CAD build for the part. Positions are in the model's coordinates, mm. A direction names the side the tool comes from. Coordinates: 2 decimals unless noted, no trailing zeros. Loops run counter-clockwise (first coordinate to the right, second up) from the corner with the lowest first, then second, coordinate; pieces in that order, holes last. Notation, with made-up numbers: M -21,0 L -4,0 A21 cw -4,4 Z; hole C 57,6.25 d5. An arc over 180 degrees is marked long. Answer as a JSON object with one key per item and string values. Group by question number.
```python
from build123d import *

# Parameters (mm, degrees)
SKETCH_1_R          = 12.2
EXTRUDE_1_DEPTH     = 18.1
FILLET_1_R          = 2
SKETCH_2_R          = 12.5
EXTRUDE_2_DEPTH     = 19
SKETCH_3_R          = 3.5
EXTRUDE_3_DEPTH     = 2.5
SKETCH_4_R          = 1.5
EXTRUDE_4_DEPTH     = 9
CUT_EXTRUDE_1_DEPTH = 8
SKETCH_6_R          = 2.25
CUT_EXTRUDE_2_DEPTH = 1.5
SKETCH_8_R          = 1.5
CUT_EXTRUDE_3_DEPTH = 6
SKETCH_9_R          = 3.25
EXTRUDE_5_DEPTH     = 2
SKETCH_10_W         = 3
SKETCH_10_H         = 0.5
EXTRUDE_6_DEPTH     = 4


with BuildPart() as part:
    # 草图1 → 凸台-拉伸1 (new body)
    with BuildSketch(Plane.XY):
        with Locations(Location((0, 0, 0), (0, 0, 180))):
            Circle(SKETCH_1_R)
    extrude(amount=EXTRUDE_1_DEPTH)

    # 圆角1
    fillet_1_edges = [part.edges().sort_by_distance(p)[0] for p in [
        (12.2, 0, 18.1),
    ]]
    fillet(fillet_1_edges, radius=FILLET_1_R)

    # 草图2 → 凸台-拉伸2 (add)
    with BuildSketch(Plane.XY.offset(18.1)):
        Circle(SKETCH_2_R)
    extrude(amount=EXTRUDE_2_DEPTH)

    # 草图3 → 凸台-拉伸3 (add)
    with BuildSketch(Plane.XY.offset(37.1)):
        Circle(SKETCH_3_R)
    extrude(amount=EXTRUDE_3_DEPTH)

    # 草图4 → 凸台-拉伸4 (add)
    with BuildSketch(Plane.XY.offset(39.6)):
        Circle(SKETCH_4_R)
    extrude(amount=EXTRUDE_4_DEPTH)

    # 草图5 → 切除-拉伸1 (cut)
    with BuildSketch(Plane.XY.offset(48.6)):
        Polygon((-1.25, -49.129490658), (-1.25, -0.829156198), (-1.25, 0.829156198), (-1.25, 49.129490658), (-97.85066892, 49.129490658), (-97.85066892, -49.129490658), align=None)
    extrude(amount=-CUT_EXTRUDE_1_DEPTH, mode=Mode.SUBTRACT)

    # 草图6 → 切除-拉伸2 (cut)
    with BuildSketch(Plane.XY.offset(37.1)):
        with Locations((8.5, 0)):
            Circle(SKETCH_6_R)
        with Locations((-8.5, 0)):
            Circle(SKETCH_6_R)
    extrude(amount=-CUT_EXTRUDE_2_DEPTH, mode=Mode.SUBTRACT)

    # 草图8 → 切除-拉伸3 (cut)
    with BuildSketch(Plane.XY.offset(37.1)):
        with Locations((0, 8.5)):
            Circle(SKETCH_8_R)
        with Locations((0, -8.5)):
            Circle(SKETCH_8_R)
    extrude(amount=-CUT_EXTRUDE_3_DEPTH, mode=Mode.SUBTRACT)

    # 草图9 → 凸台-拉伸5 (add)
    with BuildSketch(Plane(origin=(0, 0, 0), x_dir=(-1, 0, 0), z_dir=(0, 0, -1))):
        with Locations(Location((0, 0, 0), (0, 0, 180))):
            Circle(SKETCH_9_R)
    extrude(amount=EXTRUDE_5_DEPTH)

    # 草图10 → 凸台-拉伸6 (add)
    with BuildSketch(Plane(origin=(0, 0, 0), x_dir=(-1, 0, 0), z_dir=(0, 0, -1))):
        with Locations((0, 10.25)):
            Rectangle(SKETCH_10_W, SKETCH_10_H)
        with Locations((0, -10.25)):
            Rectangle(SKETCH_10_W, SKETCH_10_H)
    extrude(amount=EXTRUDE_6_DEPTH)


solid = part.part
```
Item 1: Pin check, flat tips, straight feed: pin 1 (10 mm diameter, centred on x = -7.5, y = -8, fed in from +Z); pin 2 (2 mm diameter, centred on x = 8, z = 19.5, fed in from +Y); pin 3 (4 mm diameter, centred on x = -8.5, y = 0, fed in from -Z). Stop position of each tip, or through.
Item 2: Pull direction X, two halves, no side cores. Call faces 1 (the cylindrical face through (6.252, 0.099, 36.36)), 2 (the flat face through (-1.25, 0, 45)), 3 (the cylindrical face through (11.923, 3.755, 27.467)), 4 (the flat face through (0, 0, 48.6)): released by +X, released by -X, zero draft, split by the parting line, or undercut.
Item 3: Slice it at D-D, the plane z = 24. Write the cut outline in (x, y), then the cut area to 3 significant figures.
Item 4: Slice it at B-B, the plane z = 42. Write the cut outline in (x, y).
Item 5: Drill centre lines: L1, parallel to Z at x = 0, y = -3.75; L2, parallel to X at y = 8, z = 33; L3, parallel to Z at x = 0.25, y = 7.25. Where is each one in solid material? Low to high. Write a range as from..to.
Item 6: Tool access for faces 5 (the cylindrical face through (-2.579, 1.978, -0.986)), 6 (the flat face through (0, 10, -2)), 7 (the cylindrical face through (0, 7, 34)): list every direction of +Z, -Z, +X, -X, +Y, -Y with a clear straight run to the whole face (end or side of a thin tool).
Item 7: Slice it at C-C, the plane z = 1. Write the cut outline in (x, y).
Computed:
{
 "1": {"pin 1": "z = 37.1", "pin 2": "y = 10.36", "pin 3": "z = 0"},
 "2": {"face 1": "undercut", "face 2": "released by -X", "face 3": "split by the parting line", "face 4": "zero draft"},
 "3": {"outline": "C 0,0 d25", "area": "491 mm2"},
 "4": {"outline": "M -1.25,-0.83 A1.5 ccw long -1.25,0.83 Z"},
 "5": {"L1": "0..37.1", "L2": "-9.6..-1.41, 1.41..9.6", "L3": "0..31.1"},
 "6": {"face 5": "-Z", "face 6": "-Z, +X, -X", "face 7": "+Z"},
 "7": {"outline": "C 0,0 d24.4"}
}
